Can you work these out from the model? Positions are in its coordinate system, mm. Face numbers are marked on the shaded views. Give positions to 0.01 mm unless a question says otherwise; leave off trailing zeros. Answer as CSV lines item,"result". Start each with the question number.
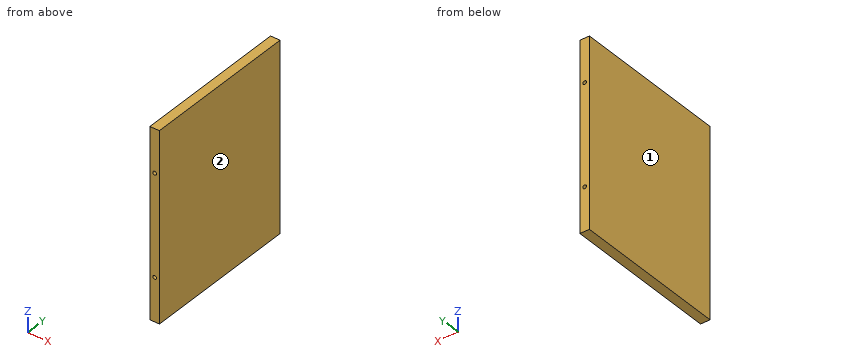
```python
from build123d import *

# Parameters (mm, degrees)
ESQUISSE1_W             = 20
ESQUISSE1_H             = 390
BOSS_EXTRU_1_DEPTH      = 330
ESQUISSE2_R             = 3.75
ENL_V_MAT_EXTRU_1_DEPTH = 10
ENL_V_START             = -10
ESQUISSE3_R             = 3.75
ENL_V_MAT_EXTRU_2_DEPTH = 10


with BuildPart() as part:
    # Esquisse1 → Boss.-Extru.1 (new body)
    with BuildSketch(Plane(origin=(0, 0, 0), x_dir=(1, 0, 0), z_dir=(0, 1, 0))):
        Rectangle(ESQUISSE1_W, ESQUISSE1_H)
    extrude(amount=BOSS_EXTRU_1_DEPTH)

    # Esquisse2 → Enlèv. mat.-Extru.1 (cut)
    with BuildSketch(Plane(origin=(0, 330, 0), x_dir=(1, 0, 0), z_dir=(0, 1, 0))):
        with Locations(Location((0, 105, 0), (0, 0, 270))):
            Circle(ESQUISSE2_R)
        with Locations(Location((0, -105, 0), (0, 0, 270))):
            Circle(ESQUISSE2_R)
    extrude(amount=-ENL_V_MAT_EXTRU_1_DEPTH, mode=Mode.SUBTRACT)

    # Esquisse3 → Enlèv. mat.-Extru.2 (cut)
    with BuildSketch(Plane.XZ.offset(ENL_V_START)):
        with Locations(Location((0, -105, 0), (0, 0, 90))):
            Circle(ESQUISSE3_R)
        with Locations(Location((0, 105, 0), (0, 0, 90))):
            Circle(ESQUISSE3_R)
    extrude(amount=ENL_V_MAT_EXTRU_2_DEPTH, mode=Mode.SUBTRACT)


solid = part.part
```
1) I'm going to push flat-ended pins straight in: P1, Ø4, axis at x = 0.5, z = 106, coming from the -Y side; P2, Ø6, axis at x = 0, z = 105, coming from the +Y side. Where does each tip first touch, or does it pass through?
2) Thinking about a two-plate mould opening in X: for the marked faces 1 and 2, which applies, released by +X, released by -X, zero draft, split by the parting line, or undercut?
3) I need wall thicknesses on L1, parallel to X at y = 7, z = -105; L2, parallel to Y at x = 1, z = -108. Which ranges of each line are inside material? Lowest first, please. Write a range as from..to.
Values found:
1,P1,"stops at y = 10"
1,P2,"stops at y = 320"
2,face 1,"released by -X"
2,face 2,"released by +X"
3,L1,"x = -10..-3.75, 3.75..10"
3,L2,"y = 10..320"
